Autodesk Inventor part; units mm, degrees
ref_plane "YZ Plane" through (0, 0, 0) normal (1, 0, 0) x (0, 1, 0)
ref_plane "XZ Plane" through (0, 0, 0) normal (0, 1, 0) x (-1, 0, 0)
ref_plane "XY Plane" through (0, 0, 0) normal (0, 0, 1) x (1, 0, 0)
sketch "Sketch1" plane through (0, 0, 0) normal (0, 0, 1) x (1, 0, 0)
  line L0 (0, 0) -> (0, 21.042)
  line L1 (0, 21.042) -> (29.758, 50.8)
  line L2 (29.758, 50.8) -> (50.8, 50.8)
  line L3 (50.8, 50.8) -> (50.8, 0)
  line L4 (50.8, 0) -> (0, 0)
  dimension "d0" = 50.8
  dimension "d2" = 50.8
  dimension "d3" = 50.8
  dimension "d4" = 135
extrude "Extrusion1" add sketch "Sketch1" along normal blind 3.175
sketch "Sketch2" plane through (0, 0, 3.175) normal (0, 0, 1) x (1, 0, 0)
  line L0 (50.8, 0) -> (50.8, 50.8)
  line L1 (0, 0) -> (50.8, 0)
  line L2 (50.8, 50.8) -> (47.625, 50.8)
  line L3 (47.625, 50.8) -> (47.625, 0)
  line L4 (47.625, 0) -> (50.8, 0)
  line L5 (50.8, 0) -> (50.8, 50.8)
  dimension "d7" = 3.175
extrude "Extrusion2" add sketch "Sketch2" against normal blind 50.8
sketch "Sketch3" plane through (50.8, 0, 3.175) normal (1, 0, 0) x (0, 0, -1)
  circle A0 centre (38.1, 36.9316) radius 3.3734
  circle A1 centre (12.7, 36.9316) radius 3.3734
  line L0 (0, 50.8) -> (50.8, 50.8)
  line L1 (0, 0) -> (0, 50.8)
  point P0 (3.175, 0)
  dimension "d10" = 6.7469
  dimension "d11" = 6.7469
  dimension "d12" = 13.8684
  dimension "d13" = 13.8684
  dimension "d14" = 12.7
  dimension "d15" = 25.4
extrude "Extrusion3" cut sketch "Sketch3" against normal blind 3.175
sketch "Sketch4" plane through (0, 0, 0) normal (0, 0, -1) x (-1, 0, 0)
  line L0 (0, 0) -> (0, 21.042)
  line L1 (0, 21.042) -> (-21.042, 0)
  line L2 (-47.625, 0) -> (0, 0)
  line L3 (0, 21.042) -> (-29.758, 50.8)
  line L4 (0, 21.042) -> (0, 0)
  line L5 (-21.042, 0) -> (0, 0)
  circle A0 centre (-20.7624, 23.8439) radius 3.3734
  circle A1 centre (-38.7229, 41.8044) radius 3.3734
  dimension "d18" = 16.6624
  dimension "d19" = 12.7
  dimension "d20" = 12.7
  dimension "d21" = 6.7469
  dimension "d22" = 25.4
extrude "Extrusion4" cut sketch "Sketch4" against normal blind 3.175
properties part number "bottom left rail gusset" material "Aluminum 6061"
The model under review builds one solid part; all positions refer to its coordinate system, in mm. A direction names the side the tool comes from. Round coordinates to 2 decimals unless told otherwise and drop trailing zeros. Order: outer loops, then holes, each group sorted by start corner. A loop starts at its lowest first (then second) coordinate and runs counter-clockwise, first axis right, second up. Notation, with made-up numbers: (36.5, 41.25) -> (60.5, 41.25) arc R11 cw to (60.5, 59.25) -> close; hole circle Ø1 at (50.25, 38.25). An arc over 180 degrees is marked (long way). One line per item, written item: value. Start each with the question number.
Q1. Wall thickness on line 1 (X direction, y = 30, z = -32) (3 decimals); line 2 (Z direction, x = 46, y = 23) (3 decimals): over which ranges is each line inside the solid? List them lowest first.
Q2. Machinability: for faces 4 (the face through (10.37, 10.67, 1.57)), 5 (the face through (29, 26, 0)), which of the approach directions +Z, -Z, +X, -X, +Y, -Y give a long, thin tool a straight path to every point of the face, cutting with its end or side? Answer none if there is none.
Q3. Take a section at A-A (z = -12). Write out the cut boundary in (x, y) (3 decimals), and give its area (3 significant figures).
Q4. Clearance check with flat-ended pins moving along their axes: pin 1 Ø8 at (y, z) = (36.93, -34.92) entering from -X (3 decimals); pin 2 Ø5 at (x, y) = (43.5, 14.5) entering from -Z. State where each tip first meets the part, or that it passes through.
Q5. Take a section at B-B (x = 19.5). Write out the cut boundary in (y, z) (3 decimals), and give its area (3 significant figures).
Q6. Mouldability with a two-part tool opening along Y and no side actions: class faces 1 (the face through (14.67, 35.71, 1.57)), 2 (the face through (47.625, 26, -23)), 3 (the face through (17.545, 24.857, 1.565)) as released by +Y, released by -Y, zero draft, split by the parting line, or undercut.
Q7. Take a section at D-D (z = -30). Write out the cut boundary in (x, y) (3 decimals).
Q8. Take a section at C-C (x = 34). Write out the cut boundary in (y, z) (3 decimals), and give its area (3 significant figures).
Reported:
1. line 1: x = 47.625 to 50.8
1. line 2: z = 0 to 3.175
2. face 4: +Z, -Z, -X, -Y
2. face 5: -Z, -X, +Y, -Y
3. outline: (47.625, 0) -> (50.8, 0) -> (50.8, 34.639) -> (47.625, 34.639) -> close; (47.625, 39.224) -> (50.8, 39.224) -> (50.8, 50.8) -> (47.625, 50.8) -> close
3. area: 147 mm2
4. pin 1: stops at x = 47.625
4. pin 2: stops at z = 0
5. outline: (1.542, 0) -> (20.716, 0) -> (20.716, 3.175) -> (1.542, 3.175) -> close; (26.972, 0) -> (40.542, 0) -> (40.542, 3.175) -> (26.972, 3.175) -> close
5. area: 104 mm2
6. face 1: released by +Y
6. face 2: zero draft
6. face 3: undercut
7. outline: (47.625, 0) -> (50.8, 0) -> (50.8, 50.8) -> (47.625, 50.8) -> close
8. outline: (0, 0) -> (50.8, 0) -> (50.8, 3.175) -> (0, 3.175) -> close
8. area: 161 mm2
